from build123d import *

# Parameters (mm, degrees)
SKETCH2_W          = 15.494
SKETCH2_H          = 15.494
CUT_EXTRUDE1_DEPTH = 12.7


with BuildPart() as part:
    # Sketch1 → Revolve1 (revolve)
    with BuildSketch(Plane.XY):
        Polygon((0, 15.875), (0, 0), (-152.4, 0), (-152.4, 19.05), (-139.7, 19.05), align=None)
    revolve(axis=Axis((0, 0, 0), (-1, 0, 0)))

    # Sketch2 → Cut-Extrude1 (cut)
    with BuildSketch(Plane(origin=(0, 0, 0), x_dir=(0, 0, -1), z_dir=(1, 0, 0))):
        Rectangle(SKETCH2_W, SKETCH2_H)
    extrude(amount=-CUT_EXTRUDE1_DEPTH, mode=Mode.SUBTRACT)


solid = part.part
Design review of the part built by this model. Coordinates are the model's own, in mm. A direction names the side the tool comes from. Coordinates: 2 decimals unless noted, no trailing zeros. Order: outer loops, then holes, each group sorted by start corner. A loop starts at its lowest first (then second) coordinate and runs counter-clockwise, first axis right, second up. Notation, with made-up numbers: (-34.5, 4.5) -> (4.5, 4.5) arc R16 cw to (4.5, 18.5) -> close; hole circle Ø1 at (47.5, 72.5). An arc over 180 degrees is marked (long way). Use one line per item in the form item = value. Start each with the question number.
(1) Add section D-D on x = -111.5. State the section outline as (y, z) points, plus the area to 3 significant figures.
(2) Add section A-A on y = 0. State the section outline as (x, z) points (3 decimals).
(3) For probe 1 along X at (y, z) = (5, 6); probe 2 along Z at (x, y) = (-106, 9); probe 3 along Y at (x, z) = (-10.5, -5.5), list the stretches that pass through material, from the lowest coordinate up.
(4) For faces 5 (the flat face through (-6, 0, -7.747)), 6 (the flat face through (-152.4, 0, 0)), list the 3-axis set-ups (+Z, -Z, +X, -X, +Y, -Y) from which the entire face can be reached by the end or side of a thin tool; tool diameter is ignored.
(5) Add section C-C on x = -27. State the section outline as (y, z) points, plus the area to 3 significant figures.
(6) Insertion check: pin 1 (4 mm diameter, centred on x = -3.5, y = 3, fed in from +Z); pin 2 (6 mm diameter, centred on x = -52, y = 14, fed in from -Z); pin 3 (3 mm diameter, centred on x = -76, z = 1.5, fed in from +Y). Each pin has a flat end and moves straight along its axis. Give the tip position at first contact, or say it passes through.
(7) The part is to be moulded in two halves that separate along Z. For faces 1 (the cylindrical face through (-145.96, -15.12, 11.59)), 2 (the flat face through (-6, 0, 7.747)), 3 (the flat face through (0, 10, 0)), 4 (the flat face through (-12.7, 0, 0)), say which applies: +Z half, -Z half, draft (parallel to the pull), parting line (faces both ways), or undercut.
Answer block:
q1.outline = circle Ø36.82 at (0, 0)
q1.area = 1,060 mm²
q2.outline = (-152.4, -19.05) -> (-139.7, -19.05) -> (0, -15.875) -> (0, -7.747) -> (-12.7, -7.747) -> (-12.7, 7.747) -> (0, 7.747) -> (0, 15.875) -> (-139.7, 19.05) -> (-152.4, 19.05) -> close
q3.probe_1 = -152.4 to -12.7
q3.probe_2 = -15.92 to 15.92
q3.probe_3 = -15.15 to -7.75, 7.75 to 15.15
q4.face_5 = +X
q4.face_6 = +Z, -Z, -X, +Y, -Y
q5.outline = circle Ø32.98 at (0, 0)
q5.area = 854 mm²
q6.pin_1 = 15.93
q6.pin_2 = -13.04
q6.pin_3 = 17.62
q7.face_1 = parting line
q7.face_2 = undercut
q7.face_3 = draft
q7.face_4 = undercut
